Input: part model. Units: mm. Frame: model coordinates. A direction names the side the tool comes from. Coordinates: 2 decimals unless noted, no trailing zeros. Order: outer loops, then holes, each group sorted by start corner. A loop starts at its lowest first (then second) coordinate and runs counter-clockwise, first axis right, second up. Notation, with made-up numbers: (-9.75, -6.5) - (27.25, -6.5) arc R17 ccw to (27.25, 21.5) - close; hole circle Ø11 at (73, 6). An arc over 180 degrees is marked (long way). One line per question, with ' | ' between items.
from build123d import *

# Parameters (mm, degrees)
SKETCH1_W                   = 88.9
SKETCH1_H                   = 25.4
BOSS_EXTRUDE1_DEPTH         = 38.1
CUT_EXTRUDE1_REACH          = 40.1
F_3_8_16_TAPPED_HOLE1_D     = 7.9375
F_1_4_20_TAPPED_HOLE1_D     = 5.1054
F_1_4_20_TAPPED_HOLE1_DEPTH = 16.51
F_1_4_20_TAPPED_HOLE1_TIP   = 1.533816902


with BuildPart() as part:
    # Sketch1 → Boss-Extrude1 (new body)
    with BuildSketch(Plane.XY):
        with Locations((0, 12.7)):
            Rectangle(SKETCH1_W, SKETCH1_H)
    extrude(amount=-BOSS_EXTRUDE1_DEPTH)

    # Sketch2 → Cut-Extrude1 (cut, up to next)
    with BuildSketch(Plane.XY, mode=Mode.PRIVATE) as cut_extrude1_sk1:
        with BuildLine():
            Line((-15.875, 25.4), (0, 25.4))
            Line((0, 25.4), (15.875, 25.4))
            Line((15.875, 25.4), (15.875, 24.13))
            Line((15.875, 24.13), (14.410694861, 24.13))
            Line((14.410694861, 24.13), (14.410694861, 22.86))
            Line((14.410694861, 22.86), (12.946389723, 22.86))
            Line((12.946389723, 22.86), (12.946389723, 21.59))
            Line((12.946389723, 21.59), (11.482084584, 21.59))
            Line((11.482084584, 21.59), (11.482084584, 20.32))
            Line((11.482084584, 20.32), (10.017779445, 20.32))
            Line((10.017779445, 20.32), (10.017779445, 19.05))
            Line((10.017779445, 19.05), (8.553474306, 19.05))
            Line((8.553474306, 19.05), (8.553474306, 17.78))
            Line((8.553474306, 17.78), (7.089169168, 17.78))
            Line((7.089169168, 17.78), (7.089169168, 16.51))
            Line((7.089169168, 16.51), (5.624864029, 16.51))
            Line((5.624864029, 16.51), (5.624864029, 15.24))
            Line((5.624864029, 15.24), (4.16055889, 15.24))
            ThreePointArc((4.16055889, 15.24), (0, 13.687108475), (-4.16055889, 15.24))
            Line((-4.16055889, 15.24), (-5.624864029, 15.24))
            Line((-5.624864029, 15.24), (-5.624864029, 16.51))
            Line((-5.624864029, 16.51), (-7.089169168, 16.51))
            Line((-7.089169168, 16.51), (-7.089169168, 17.78))
            Line((-7.089169168, 17.78), (-8.553474306, 17.78))
            Line((-8.553474306, 17.78), (-8.553474306, 19.05))
            Line((-8.553474306, 19.05), (-10.017779445, 19.05))
            Line((-10.017779445, 19.05), (-10.017779445, 20.32))
            Line((-10.017779445, 20.32), (-11.482084584, 20.32))
            Line((-11.482084584, 20.32), (-11.482084584, 21.59))
            Line((-11.482084584, 21.59), (-12.946389723, 21.59))
            Line((-12.946389723, 21.59), (-12.946389723, 22.86))
            Line((-12.946389723, 22.86), (-14.410694861, 22.86))
            Line((-14.410694861, 22.86), (-14.410694861, 24.13))
            Line((-14.410694861, 24.13), (-15.875, 24.13))
            Line((-15.875, 24.13), (-15.875, 25.4))
        make_face()
    cut_extrude1_tool1 = extrude(cut_extrude1_sk1.sketch, amount=-CUT_EXTRUDE1_REACH, mode=Mode.PRIVATE) & part.part
    add(cut_extrude1_tool1.solids().sort_by_distance((0, 20.970592, 0))[0], mode=Mode.SUBTRACT)

    # 3/8-16 Tapped Hole1 (through all)
    with Locations(Plane(origin=(0, 25.4, 0), x_dir=(1, 0, 0), z_dir=(0, 1, 0))):
        with Locations((-31.75, 19.05), (31.75, 19.05)):
            Hole(F_3_8_16_TAPPED_HOLE1_D / 2)

    # 1/4-20 Tapped Hole1
    with Locations(Plane(origin=(0, 0, 0), x_dir=(-1, 0, 0), z_dir=(0, -1, 0))):
        with Locations((-20.32, 19.05), (20.32, 19.05)):
            Hole(F_1_4_20_TAPPED_HOLE1_D / 2, depth=F_1_4_20_TAPPED_HOLE1_DEPTH)
            with Locations((0, 0, -(F_1_4_20_TAPPED_HOLE1_DEPTH + F_1_4_20_TAPPED_HOLE1_TIP / 2))):  # 118° drill point
                Cone(0, F_1_4_20_TAPPED_HOLE1_D / 2, F_1_4_20_TAPPED_HOLE1_TIP, mode=Mode.SUBTRACT)


solid = part.part
Item 1: Section B-B on y = 8. Return the cut outline in (x, z).
Data:
outline: (-44.45, -38.1) - (44.45, -38.1) - (44.45, 0) - (-44.45, 0) - close; hole circle Ø7.94 at (-31.75, -19.05); hole circle Ø5.11 at (-20.32, -19.05); hole circle Ø5.11 at (20.32, -19.05); hole circle Ø7.94 at (31.75, -19.05)
Item 2: Ray query, line 1 (X direction, y = 18.5, z = -19.05); line 2 (X direction, y = 11.5, z = -19.05); line 3 (X direction, y = 21.25, z = -35). Return the intervals inside material, ascending.
Data:
line 1: -44.45 to -35.72, -27.78 to -8.55, 8.55 to 27.78, 35.72 to 44.45 | line 2: -44.45 to -35.72, -27.78 to -22.87, -17.77 to 17.77, 22.87 to 27.78, 35.72 to 44.45 | line 3: -44.45 to -11.48, 11.48 to 44.45
Item 3: Section A-A on x = -31.75. Return the cut outline in (y, z), and give its area (3 significant figures).
Data:
outline: (0, -38.1) - (25.4, -38.1) - (25.4, -23.02) - (0, -23.02) - close; (0, -15.08) - (25.4, -15.08) - (25.4, 0) - (0, 0) - close | area: 766 mm^2
Item 4: Contact query for flat-ended pins moving along their axis: P1, Ø1.2, axis at x = 6, z = -20.5, coming from the +Y side; P2, Ø8, axis at x = 8, z = -17, coming from the +Y side; P3, Ø0.7, axis at x = 15, z = -25, coming from the +Y side; P4, Ø2, axis at x = 11, z = -7.5, coming from the -Y side. Output: stop coordinate, or through.
Data:
P1: y = 16.51 | P2: y = 21.59 | P3: y = 24.13 | P4: y = 0
Item 5: Access query for faces 1 (the face through (-19.142, 8.371, -16.785)), 2 (the face through (-28.825, 12.522, -21.732)). Directions: +Z, -Z, +X, -X, +Y, -Y. A direction counts if a zero-diameter tool reaches every point of the face in a straight line with its end or side. Return the directions, or none.
Data:
face 1: -Y | face 2: +Y, -Y
Item 6: Draft query along X for faces 3 (the face through (0.064, 13.687, -18.783)), 4 (the face through (44.45, 13, -19)), 5 (the face through (-1, 13, 0)), 6 (the face through (34.675, 12.522, -21.732)). Return one class per face: released by +X, released by -X, zero draft, split by the parting line, or undercut.
Data:
face 3: undercut | face 4: released by +X | face 5: zero draft | face 6: undercut
